from build123d import *

# Parameters (mm, degrees)
F0_R     = 5
F1_DEPTH = 12
F2_R     = 2.5
F3_DEPTH = 25
F4_R     = 2.5
F5_DEPTH = 25


with BuildPart() as f1:
    # F0 (on Right) → F1 (new body)
    with BuildSketch(Plane.YZ):
        with BuildLine():
            Line((-60, 120), (-60, 0))
            Line((-60, 0), (60, 0))
            Line((60, 0), (60, 140))
            Line((60, 140), (-40, 140))
            ThreePointArc((-40, 140), (-54.142136, 134.142136), (-60, 120))
        make_face()
        with Locations((-30, 9)):
            Circle(F0_R, mode=Mode.SUBTRACT)
        with Locations((30, 9)):
            Circle(F0_R, mode=Mode.SUBTRACT)
        with Locations((51, 30)):
            Circle(F0_R, mode=Mode.SUBTRACT)
        with BuildLine():
            Line((-48, 82.5), (-48, 117.5))
            ThreePointArc((-48, 117.5), (-46.535534, 121.035534), (-43, 122.5))
            ThreePointArc((-43, 122.5), (-39.464466, 121.035534), (-38, 117.5))
            Line((-38, 117.5), (-38, 82.5))
            ThreePointArc((-38, 82.5), (-39.464466, 78.964466), (-43, 77.5))
            ThreePointArc((-43, 77.5), (-46.535534, 78.964466), (-48, 82.5))
        make_face(mode=Mode.SUBTRACT)
        with Locations((51, 110)):
            Circle(F0_R, mode=Mode.SUBTRACT)
    extrude(amount=F1_DEPTH)

    # F2 (on face) → F3 (cut)
    with BuildSketch(Plane(origin=(0, 0, 0), x_dir=(1, 0, 0), z_dir=(0, 0, -1))):
        with Locations((6, 0)):
            Circle(F2_R)
        with Locations((6, 30)):
            Circle(F2_R)
        with Locations((6, -30)):
            Circle(F2_R)
    extrude(amount=-F3_DEPTH, mode=Mode.SUBTRACT)

    # F4 (on face) → F5 (cut)
    with BuildSketch(Plane(origin=(0, 60, 0), x_dir=(-1, 0, 0), z_dir=(0, 1, 0))):
        with Locations((-6, 70)):
            Circle(F4_R)
        with Locations((-6, 110)):
            Circle(F4_R)
        with Locations((-6, 30)):
            Circle(F4_R)
    extrude(amount=-F5_DEPTH, mode=Mode.SUBTRACT)


solid = f1.part
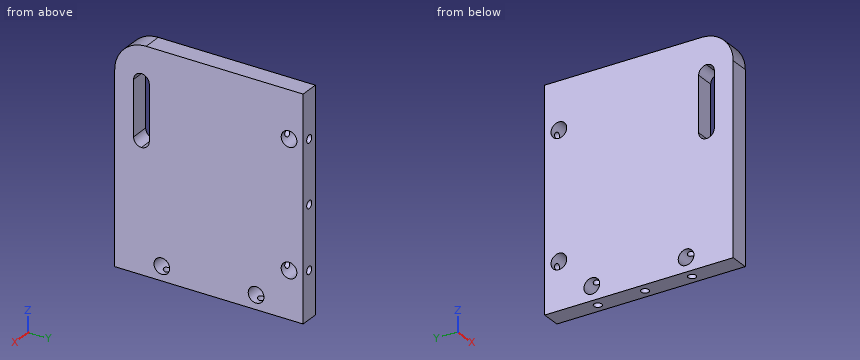
Can you work these out from the model? Positions are in its coordinate system, mm. Give positions to 0.01 mm unless a question says otherwise; leave off trailing zeros. Loops run counter-clockwise (first coordinate to the right, second up) from the corner with the lowest first, then second, coordinate; pieces in that order, holes last. Notation, with made-up numbers: (75.5, -20.5) -> (123.5, -20.5) arc R20 cw to (123.5, 11.5) -> close; hole circle Ø1 at (10.25, 0). An arc over 180 degrees is marked (long way). Write item = value, one per line.
1) I need wall thicknesses on L1, parallel to Y at x = 6, z = 1.95; L2, parallel to Z at x = 6, y = 58.7; L3, parallel to X at y = 30, z = 1. Which ranges of each line are inside material? Lowest first, please. Write a range as from..to.
Check result:
L1 = -60..-32.5, -27.5..-2.5, 2.5..27.5, 32.5..60
L2 = 0..27.5, 32.5..67.5, 72.5..107.5, 112.5..140
L3 = 0..3.5, 8.5..12
2) Will these pins go through, and if not, where does the flat tip stop? pin 1 (1.5 mm diameter, centred on x = 5, z = 111, fed in from +Y); pin 2 (1.5 mm diameter, centred on x = 5.5, y = -0.5, fed in from -Z).
Check result:
pin_1 = 35
pin_2 = 25
3) Suppose I cut it at A-A on z = 9. Write out the boundary of the cut face in (x, y), then the cut area to 3 significant figures.
Check result:
outline = (0, -60) -> (12, -60) -> (12, -35) -> (0, -35) -> close; (0, -25) -> (12, -25) -> (12, 25) -> (0, 25) -> close; (0, 35) -> (12, 35) -> (12, 60) -> (0, 60) -> close; hole circle Ø5 at (6, 0)
area = 1,180 mm2
4) Suppose I cut it at C-C on z = 30. Write out the boundary of the cut face in (x, y), then the cut area to 4 significant figures.
Check result:
outline = (0, -60) -> (12, -60) -> (12, 46) -> (8.5, 46) -> (8.5, 35) -> (3.5, 35) -> (3.5, 46) -> (0, 46) -> close; (0, 56) -> (3.5, 56) -> (3.5, 60) -> (0, 60) -> close; (8.5, 56) -> (12, 56) -> (12, 60) -> (8.5, 60) -> close
area = 1,245 mm2
5) Suppose I cut it at B-B on y = 30. Write out the boundary of the cut face in (x, z), then the cut area to 4 significant figures.
Check result:
outline = (0, 0) -> (3.5, 0) -> (3.5, 4) -> (0, 4) -> close; (0, 14) -> (3.5, 14) -> (3.5, 25) -> (8.5, 25) -> (8.5, 14) -> (12, 14) -> (12, 140) -> (0, 140) -> close; (8.5, 0) -> (12, 0) -> (12, 4) -> (8.5, 4) -> close
area = 1,485 mm2
6) Suppose I cut it at D-D on y = 51. Write out the boundary of the cut face in (x, z), then the cut area to 3 significant figures.
Check result:
outline = (0, 0) -> (12, 0) -> (12, 25) -> (0, 25) -> close; (0, 35) -> (12, 35) -> (12, 105) -> (0, 105) -> close; (0, 115) -> (12, 115) -> (12, 140) -> (0, 140) -> close; hole circle Ø5 at (6, 70)
area = 1,420 mm2
